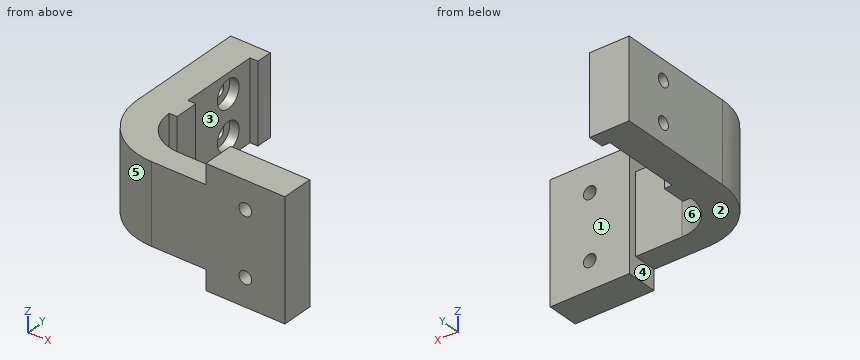
```python
from build123d import *

# Parameters (mm, degrees)
BOSS_EXTRUDE1_DEPTH         = 5
TAP_DRILL_FOR_M2X0_4_TAP1_D = 1.6
SKETCH4_R                   = 1.75
CUT_EXTRUDE1_DEPTH          = 1.2
SKETCH5_W                   = 10
SKETCH5_H                   = 15
BOSS_EXTRUDE2_DEPTH         = 4
TAP_DRILL_FOR_M2X0_4_TAP2_D = 1.6


with BuildPart() as part:
    # Sketch1 → Boss-Extrude1 (new, symmetric)
    with BuildSketch(Plane.XY):
        with BuildLine():
            Line((-17.53737418, 3), (-17.53737418, 13))
            Line((-17.53737418, 13), (-16.53737418, 13))
            Line((-16.53737418, 13), (-16.53737418, 15))
            Line((-16.53737418, 15), (-21.53737418, 15))
            Line((-21.53737418, 15), (-21.53737418, 0))
            ThreePointArc((-21.53737418, 0), (-19.162010175, -5.734635995), (-13.42737418, -8.11))
            Line((-13.42737418, -8.11), (3.46262582, -8.11))
            Line((3.46262582, -8.11), (3.46262582, -5.11))
            Line((3.46262582, -5.11), (-12.42737418, -5.11))
            ThreePointArc((-12.42737418, -5.11), (-16.040689832, -3.613315652), (-17.53737418, 0))
            Line((-17.53737418, 0), (-16.53737418, 0))
            Line((-16.53737418, 0), (-16.53737418, 3))
            Line((-16.53737418, 3), (-17.53737418, 3))
        make_face()
    extrude(amount=BOSS_EXTRUDE1_DEPTH, both=True)

    # Tap Drill for M2x0.4 Tap1 (through all)
    with Locations(Plane(origin=(-17.53737418, 9.5, 2.5), x_dir=(0, 0, 1), z_dir=(1, 0, 0))):
        with Locations((0, 0), (-5, 0)):
            Hole(TAP_DRILL_FOR_M2X0_4_TAP1_D / 2)

    # Sketch4 → Cut-Extrude1 (cut)
    with BuildSketch(Plane(origin=(-17.53737418, 0, 0), x_dir=(0, 0, -1), z_dir=(1, 0, 0))):
        with Locations((-2.5, 9.5)):
            Circle(SKETCH4_R)
        with Locations((2.5, 9.5)):
            Circle(SKETCH4_R)
    extrude(amount=-CUT_EXTRUDE1_DEPTH, mode=Mode.SUBTRACT)

    # Sketch5 → Boss-Extrude2 (add)
    with BuildSketch(Plane.XZ.offset(8.11)):
        with Locations((-1.53737418, 0)):
            Rectangle(SKETCH5_W, SKETCH5_H)
    extrude(amount=-BOSS_EXTRUDE2_DEPTH)

    # Tap Drill for M2x0.4 Tap2 (through all)
    with Locations(Plane(origin=(-1.53737418, -4.11, 4), x_dir=(0, 0, 1), z_dir=(0, 1, 0))):
        with Locations((0, 0), (-8, 0)):
            Hole(TAP_DRILL_FOR_M2X0_4_TAP2_D / 2)


solid = part.part
```
Here's how the part is built. I have some questions about the finished solid (model axes, mm). Face numbers are marked on the shaded views. A direction names the side the tool comes from. Coordinates: 2 decimals unless noted, no trailing zeros. Loops run counter-clockwise (first coordinate to the right, second up) from the corner with the lowest first, then second, coordinate; pieces in that order, holes last. Notation, with made-up numbers: (-35.75, 2) -> (-14.75, 2) arc R25 cw to (-14.75, 24) -> close; hole circle Ø5 at (79, 10). An arc over 180 degrees is marked (long way). Return JSON: item names as keys, results as strings.
1) If we section it at C-C, the plane y = -6: Write out the boundary of the cut face in (x, z).
Results below:
{"outline": "(-18.88, -5) -> (-6.54, -5) -> (-6.54, -7.5) -> (3.46, -7.5) -> (3.46, 7.5) -> (-6.54, 7.5) -> (-6.54, 5) -> (-18.88, 5) -> close; hole circle Ø1.6 at (-1.54, -4); hole circle Ø1.6 at (-1.54, 4)"}
2) For the marked faces 1, 2 and 3, which set-ups out of +Z, -Z, +X, -X, +Y, -Y let a thin tool reach every point of the face, with its end or its side?
Results below:
{"face 1": "+Z, -Z, +X, +Y", "face 2": "-Z, -X, +Y, -Y", "face 3": "+Z, -Z, +X"}
3) Thinking about a two-plate mould opening in Y: for the marked faces 4, 5 and 6, which applies, +Y half, -Y half, draft (parallel to the pull), parting line (faces both ways), or undercut?
Results below:
{"face 4": "draft", "face 5": "-Y half", "face 6": "undercut"}
4) If we section it at D-D, the plane z = -2.75: Write out the boundary of the cut face in (x, y).
Results below:
{"outline": "(-21.54, 0) arc R8.11 ccw to (-13.43, -8.11) -> (3.46, -8.11) -> (3.46, -4.11) -> (-6.54, -4.11) -> (-6.54, -5.11) -> (-12.43, -5.11) arc R5.11 cw to (-17.54, 0) -> (-16.54, 0) -> (-16.54, 3) -> (-17.54, 3) -> (-17.54, 7.77) -> (-18.74, 7.77) -> (-18.74, 8.74) -> (-21.54, 8.74) -> close; (-21.54, 10.26) -> (-18.74, 10.26) -> (-18.74, 11.23) -> (-17.54, 11.23) -> (-17.54, 13) -> (-16.54, 13) -> (-16.54, 15) -> (-21.54, 15) -> close"}
5) If we section it at A-A, the plane y = 9.5: Write out the boundary of the cut face in (x, z).
Results below:
{"outline": "(-21.54, -5) -> (-17.54, -5) -> (-17.54, -4.25) -> (-18.74, -4.25) -> (-18.74, -3.3) -> (-21.54, -3.3) -> close; (-21.54, -1.7) -> (-18.74, -1.7) -> (-18.74, -0.75) -> (-17.54, -0.75) -> (-17.54, 0.75) -> (-18.74, 0.75) -> (-18.74, 1.7) -> (-21.54, 1.7) -> close; (-21.54, 3.3) -> (-18.74, 3.3) -> (-18.74, 4.25) -> (-17.54, 4.25) -> (-17.54, 5) -> (-21.54, 5) -> close"}
6) Will these pins go through, and if not, where does the flat tip stop? pin 1 (4.5 mm diameter, centred on y = -5.5, z = 1, fed in from -X); pin 2 (2 mm diameter, centred on y = 14, z = 0.5, fed in from +X); pin 3 (5 mm diameter, centred on y = 10.5, z = -5.5, fed in from +X).
Results below:
{"pin 1": "x = -20.86", "pin 2": "x = -16.54", "pin 3": "x = -17.54"}
7) I need wall thicknesses on line 1 (Z direction, x = -19.6, y = 9.5); line 2 (Y direction, x = -17, z = 2); line 3 (Y direction, x = -6.25, z = 6.25). Which ranges of each line are inside material? Lowest first, please. Write a range as from..to.
Results below:
{"line 1": "-5..-3.3, -1.7..1.7, 3.3..5", "line 2": "-7.28..-2.28, 0..3, 13..15", "line 3": "-8.11..-4.11"}
8) If we section it at B-B, the plane z = 2.5: Write out the boundary of the cut face in (x, y), then the cut area to 3 significant figures.
Results below:
{"outline": "(-21.54, 0) arc R8.11 ccw to (-13.43, -8.11) -> (3.46, -8.11) -> (3.46, -4.11) -> (-6.54, -4.11) -> (-6.54, -5.11) -> (-12.43, -5.11) arc R5.11 cw to (-17.54, 0) -> (-16.54, 0) -> (-16.54, 3) -> (-17.54, 3) -> (-17.54, 7.75) -> (-18.74, 7.75) -> (-18.74, 8.7) -> (-21.54, 8.7) -> close; (-21.54, 10.3) -> (-18.74, 10.3) -> (-18.74, 11.25) -> (-17.54, 11.25) -> (-17.54, 13) -> (-16.54, 13) -> (-16.54, 15) -> (-21.54, 15) -> close", "area": "153 mm²"}
